```python
from build123d import *

# Parameters (mm, degrees)
SKETCH1_W           = 152.4
SKETCH1_H           = 12.7
BOSS_EXTRUDE1_DEPTH = 6.35
FILLET1_R           = 6.35
SKETCH2_R           = 2.38125
CUT_EXTRUDE1_DEPTH  = 25.4


with BuildPart() as part:
    # Sketch1 → Boss-Extrude1 (new body)
    with BuildSketch(Plane.XY):
        with Locations((76.2, 6.35)):
            Rectangle(SKETCH1_W, SKETCH1_H)
    extrude(amount=BOSS_EXTRUDE1_DEPTH)

    # Fillet1
    fillet1_edges = [part.edges().sort_by_distance(p)[0] for p in [
        (0, 0, 3.175),
        (0, 12.7, 3.175),
        (152.4, 0, 3.175),
        (152.4, 12.7, 3.175),
    ]]
    fillet(fillet1_edges, radius=FILLET1_R - 0.0001)  # a hair under: the kernel refuses the full size

    # Sketch2 → Cut-Extrude1 (cut)
    with BuildSketch(Plane.XY.offset(6.35)):
        with Locations((6.35, 6.35)):
            Circle(SKETCH2_R)
        with Locations((146.05, 6.35)):
            Circle(SKETCH2_R)
    extrude(amount=-CUT_EXTRUDE1_DEPTH, mode=Mode.SUBTRACT)


solid = part.part
```
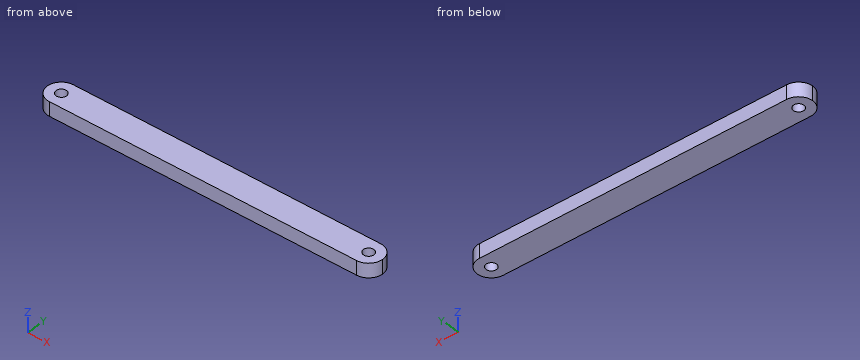
Can you work these out from the model? Positions are in its coordinate system, mm. Round coordinates to 2 decimals unless told otherwise and drop trailing zeros. Order: outer loops, then holes, each group sorted by start corner. A loop starts at its lowest first (then second) coordinate and runs counter-clockwise, first axis right, second up. Notation, with made-up numbers: (-1.5, 86.5) -> (35.5, 86.5) arc R18 ccw to (35.5, 96.5) -> close; hole circle Ø2 at (-29, 46). An arc over 180 degrees is marked (long way). Return JSON: item names as keys, results as strings. Group by question number.
1. If we section it at A-A, the plane z = 4.5: Count the separate pieces of the cut face and the enclosed holes in it, then the cut area to 3 significant figures.
2. If we section it at C-C, the plane y = 2: Write out the boundary of the cut face in (x, z).
3. I need wall thicknesses on line 1 (X direction, y = 6, z = 3.5); line 2 (Y direction, x = 6.35, z = 1.75); line 3 (X direction, y = 8.5, z = 4). Which ranges of each line are inside material? Lowest first, please. Write a range as [from, to].
4. If we section it at B-B, the plane y = 10.5: Write out the boundary of the cut face in (x, z), then the cut area to 3 significant figures.
Output values:
{
 "1": {"separate pieces": "1", "enclosed holes": "2", "area": "1,870 mm²"},
 "2": {"outline": "(1.72, 0) -> (150.68, 0) -> (150.68, 6.35) -> (1.72, 6.35) -> close"},
 "3": {"line 1": "[0.01, 3.99], [8.71, 143.69], [148.41, 152.39]", "line 2": "[0, 3.97], [8.73, 12.7]", "line 3": "[0.38, 5.33], [7.37, 145.03], [147.07, 152.02]"},
 "4": {"outline": "(1.54, 0) -> (150.86, 0) -> (150.86, 6.35) -> (1.54, 6.35) -> close", "area": "948 mm²"}
}
